```python
from build123d import *

# Parameters (mm, degrees)
SKETCH1_W               = 101.6
SKETCH1_H               = 50.8
BOSS_EXTRUDE1_DEPTH     = 331.365720046
CUT_EXTRUDE1_DEPTH      = 340.064183336
CUT_EXTRUDE1_DEPTH_BACK = 340.064183336
CUT_EXTRUDE2_DEPTH      = 340.064183336
CUT_EXTRUDE2_DEPTH_BACK = 340.064183336
SKETCH3_W               = 12.7
SKETCH3_H               = 355.6


with BuildPart() as part:
    # Sketch1 → Boss-Extrude1 (new body)
    with BuildSketch(Plane.XY):
        Rectangle(SKETCH1_W, SKETCH1_H)
    extrude(amount=BOSS_EXTRUDE1_DEPTH)

    # Sketch2 → Cut-Extrude1 (cut, two sides: drawn at the far end of the back side and taken through both)
    with BuildSketch(Plane(origin=(0, 25.4, 0), x_dir=(1, 0, 0), z_dir=(0, 1, 0)).offset(-CUT_EXTRUDE1_DEPTH_BACK)):
        Polygon((50.8, -324.424970201), (1.413998706, -331.365720046), (50.8, -331.365720046), align=None)
        Polygon((0, -321.304596468), (-50.8, -328.44407087), (-50.8, -331.365720046), (1.413998706, -331.365720046), align=None)
    extrude(amount=CUT_EXTRUDE1_DEPTH + CUT_EXTRUDE1_DEPTH_BACK, mode=Mode.SUBTRACT)

    # Sketch3 → Cut-Extrude2 (cut, two sides: drawn at the far end of the back side and taken through both)
    with BuildSketch(Plane.XZ.offset(25.4).offset(-CUT_EXTRUDE2_DEPTH_BACK)):
        with Locations((44.45, 177.8)):
            Rectangle(SKETCH3_W, SKETCH3_H)
    extrude(amount=CUT_EXTRUDE2_DEPTH + CUT_EXTRUDE2_DEPTH_BACK, mode=Mode.SUBTRACT)


solid = part.part
```
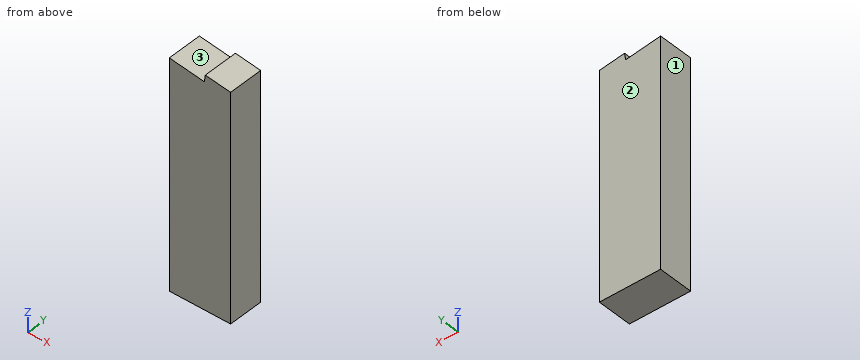
Work out the finished part from the listing and answer in its coordinate system (mm). Face numbers are marked on the shaded views. Give positions to 0.01 mm unless a question says otherwise; leave off trailing zeros. Loops run counter-clockwise (first coordinate to the right, second up) from the corner with the lowest first, then second, coordinate; pieces in that order, holes last. Notation, with made-up numbers: (33.25, 61) - (49.25, 61) arc R26 cw to (49.25, 87) - close; hole circle Ø11 at (-33.75, -20.75). An arc over 180 degrees is marked (long way). Use CSV: the item, a comma, the result in double quotes. Start each with the question number.
(1) Find section A-A, the plane x = -34.5. Determine the outline of the cut face in (y, z), plus the area to 3 significant figures.
(2) Find the intervals of material crossed by L1, parallel to Z at x = -35, y = -2.5; L2, parallel to Z at x = -32, y = -6, in increasing order.
(3) Determine the mould class of the marked faces 1, 2 and 3 for opening direction X: released by +X, released by -X, zero draft, split by the parting line, or undercut.
Results found:
1,outline,"(-25.4, 0) - (25.4, 0) - (25.4, 326.15) - (-25.4, 326.15) - close"
1,area,"16,600 mm^2"
2,L1,"0 to 326.22"
2,L2,"0 to 325.8"
3,face 1,"released by -X"
3,face 2,"zero draft"
3,face 3,"undercut"
